For this review, take the finished solid that the model builds, in its own axes (mm). A direction names the side the tool comes from. Round coordinates to 2 decimals unless told otherwise and drop trailing zeros. Loops run counter-clockwise (first coordinate to the right, second up) from the corner with the lowest first, then second, coordinate; pieces in that order, holes last.
Autodesk Inventor part; units mm, degrees
ref_plane "Work Plane2" through (-2.5, 0, 0) normal (1, 0, 0) x (0, 1, 0)
ref_plane "Work Plane3" through (-15, 0, 0) normal (1, 0, 0) x (0, 1, 0)
ref_plane "XZ Plane" through (0, 0, 0) normal (0, 1, 0) x (-1, 0, 0)
sketch "Sketch1" plane through (0, 0, 0) normal (0, 1, 0) x (-1, 0, 0)
  line L0 (0, 0) -> (30, 0)
  line L1 (30, 0) -> (30, -10)
  line L2 (30, -10) -> (0, -10)
  line L3 (0, -10) -> (0, 0)
  dimension "d0" = 30
  dimension "d1" = 10
extrude "Extrusion1" add sketch "Sketch1" along normal blind 3
ref_plane "Work Plane2" through (-2.5, 0, 0) normal (1, 0, 0) x (0, 1, 0)
sketch "Sketch3" plane through (-2.5, 0, 0) normal (1, 0, 0) x (0, 1, 0)
  line L0 (3, -10) -> (3, 0)
  line L1 (3, 0) -> (10, 7)
  line L2 (10, 7) -> (10, 13.5)
  line L3 (10, 13.5) -> (0, 4)
  line L4 (0, 4) -> (0, 0)
  line L5 (0, 0) -> (3, 0)
  line L6 (3, 0) -> (0, 0)
  dimension "d13" = 4
  dimension "d14" = 6.5
  dimension "d15" = 45
  dimension "d16" = 10
extrude "Extrusion3" add sketch "Sketch3" against normal blind 5
ref_plane "Work Plane3" through (-15, 0, 0) normal (1, 0, 0) x (0, 1, 0)
fillet "Fillet2" radius 2 1 edges at (-5, 0, 4)
fillet "Fillet3" radius 2 4 edges at (-30, 1.5, 0) (-7.5, 1.5, 0) (-2.5, 1.5, 0) (0, 1.5, 0)
fillet "Fillet4" radius 5 2 edges at (-30, 1.5, -10) (0, 1.5, -10)
sketch "Sketch5" plane through (-2.5, 10, 13.5) normal (0, 1, 0) x (1, 0, 0)
  line L0 (-1.1, 5.4) -> (-3.9, 5.4)
  line L1 (-3.9, 5.4) -> (-3.9, 1.1)
  line L2 (-3.9, 1.1) -> (-1.1, 1.1)
  line L3 (-1.1, 1.1) -> (-1.1, 5.4)
  line L4 (-5, 0) -> (-5, 6.5)
  line L5 (0, 6.5) -> (-5, 6.5)
  point P0 (2.5, 13.5)
  dimension "d26" = 2.8
  dimension "d27" = 4.3
  dimension "d28" = 1.1
  dimension "d29" = 1.1
extrude "Extrusion4" add sketch "Sketch5" along normal blind 2
mirror "Mirror2" about plane through (-15, 0, 0) normal (1, 0, 0) of "Extrusion3", "Extrusion4"
sketch "Sketch6" plane through (0, 3, 0) normal (0, 1, 0) x (1, 0, 0)
  circle A0 centre (-15, 5) radius 3
  line L0 (-5, 10) -> (-25, 10)
  line L1 (0, 1.7081) -> (0, 5)
  point P0 (0, 0)
  dimension "d32" = 6
  dimension "d33" = 5
  dimension "d34" = 15
extrude "Extrusion5" cut sketch "Sketch6" against normal through all
chamfer "Chamfer1" distance 1 angle 45 1 edges at (-18, 3, -5)
sketch "Sketch7" plane through (0, 3, 0) normal (0, 1, 0) x (1, 0, 0)
  circle A0 centre (-23, 5) radius 1
  circle A1 centre (-7, 5) radius 1
  line L0 (-5, 10) -> (-25, 10)
  circle A2 centre (-15, 5) radius 3
  point P0 (0, 0)
  dimension "d40" = 2
  dimension "d41" = 2
  dimension "d42" = 5
  dimension "d43" = 5
  dimension "d44" = 8
  dimension "d45" = 8
extrude "Extrusion6" cut sketch "Sketch7" against normal through all contours A0 | A1
chamfer "Chamfer2" distance 1 angle 45 2 edges at (-8, 3, -5) (-24, 3, -5)
fillet "Fillet5" radius 2 1 edges at (-25, 0, 4)
chamfer "Chamfer3" distance 1 angle 45 1 edges at (-18, 0, -5)
properties part number "ServoUltrasonicMount"
(1) Insertion check: pin 1 Ø2 at (x, y) = (-24.5, 11.5) entering from +Z; pin 2 Ø5 at (x, z) = (-3.5, 3) entering from +Y; pin 3 Ø1 at (x, y) = (-5.5, 11) entering from -Z. Each pin has a flat end and moves straight along its axis. Give the tip position at first contact, or say it passes through.
(2) Add section D-D (x = -7). Give the boundary of the cut face in (y, z), plus the area to 3 significant figures.
(3) Add section A-A (x = -15). Give the boundary of the cut face in (y, z).
(4) For L1, parallel to X at y = 1.6, z = -5; L2, parallel to X at y = 9, z = 8.5; L3, parallel to Z at x = -15, y = 1.8, list the stretches that pass through material, from the lowest coordinate up.
(5) For faces 4 (the flat face through (-14.8, 0, -0.4)), 5 (the flat face through (-22.5, 5, 5)), 6 (the flat face through (-2.5, 6, 7)), 7 (the flat face through (-23.6, 11, 10)), 8 (the flat face through (-27.5, 5, 5)), list the 3-axis set-ups (+Z, -Z, +X, -X, +Y, -Y) from which the entire face can be reached by the end or side of a thin tool; tool diameter is ignored.
(6) Add section C-C (y = 6.25). Give the boundary of the cut face in (x, z).
(7) Add section B-B (z = 9.25). Give the boundary of the cut face in (x, y).
(8) The part is to be moulded in two halves that separate along X. For faces 1 (the flat face through (-26.4, 11, 10)), 2 (the flat face through (-3.6, 11, 10)), 3 (the cylindrical face through (-17.4, 1.5, -3.2)), say which applies: pulls with the +X half, pulls with the -X half, needs draft (parallel to the pull), parting line crosses it, or undercut.
Outcome:
1. pin 1: stops at z = 12.4
1. pin 2: stops at y = 8.5
1. pin 3: stops at z = 8.1
2. outline: (0, -10) - (3, -10) - (3, -7) - (2, -6) - (0, -6) - close; (0, -4) - (2, -4) - (3, -3) - (3, 0) - (10, 7) - (10, 13.5) - (0.62, 4.59) arc R2 ccw to (0, 3.14) - close
2. area: 85.9 mm2
3. outline: (0, -10) - (3, -10) - (3, -9) - (2, -8) - (1, -8) - (0, -9) - close; (0, -1) - (1, -2) - (2, -2) - (3, -1) - (3, 0) - (0, 0) - close
4. L1: x = -30 to -24, -22 to -18, -12 to -8, -6 to 0
4. L2: x = -27.5 to -22.5, -7.5 to -2.5
4. L3: z = -10 to -8, -2 to 0
5. face 4: +Z, -Z, +X, -X, -Y
5. face 5: +Z, +Y, -Y
5. face 6: +Z, +X, +Y, -Y
5. face 7: +Z, -Z, +Y
5. face 8: +Z, -X, +Y, -Y
6. outline: (-27.5, 3.25) - (-22.5, 3.25) - (-22.5, 9.94) - (-27.5, 9.94) - close; (-7.5, 3.25) - (-2.5, 3.25) - (-2.5, 9.94) - (-7.5, 9.94) - close
7. outline: (-27.5, 5.53) - (-22.5, 5.53) - (-22.5, 10) - (-23.6, 10) - (-23.6, 12) - (-26.4, 12) - (-26.4, 10) - (-27.5, 10) - close; (-7.5, 5.53) - (-2.5, 5.53) - (-2.5, 10) - (-3.6, 10) - (-3.6, 12) - (-6.4, 12) - (-6.4, 10) - (-7.5, 10) - close
8. face 1: pulls with the -X half
8. face 2: pulls with the +X half
8. face 3: undercut
